from build123d import *

# Parameters (mm, degrees)
ESBO_O1_W                  = 44
ESBO_O1_H                  = 44
RESSALTO_EXTRUS_O1_DEPTH   = 12
ESBO_O2_R                  = 18
RESSALTO_EXTRUS_O2_DEPTH   = 17
CHANFRO1_SIZE              = 7
CORTE_EXTRUS_O1_DEPTH      = 1
CORTE_EXTRUS_O1_DEPTH_BACK = 43.532340636
ESBO_O3_R                  = 6
ESBO_O3_R_2                = 2.5
ESBO_O4_R                  = 4
CORTE_EXTRUS_O2_DEPTH      = 5
CHANFRO2_SIZE              = 0.5
CHANFRO3_SIZE              = 0.5
ESBO_O5_R                  = 7.5
ESBO_O5_R_2                = 7.25
CORTE_EXTRUS_O3_DEPTH      = 1
ESBO_O6_R                  = 8.146724453
ESBO_O6_R_2                = 7.952420513
CORTE_EXTRUS_O4_DEPTH      = 1
ESBO_O7_R                  = 12.470388764
ESBO_O7_R_2                = 11.825568989
CORTE_EXTRUS_O5_DEPTH      = 1
FILETE1_R                  = 0.2
FILETE2_R                  = 0.2


with BuildPart() as part:
    # Esboço1 → Ressalto-extrusão1 (new body)
    with BuildSketch(Plane.XY):
        Rectangle(ESBO_O1_W, ESBO_O1_H)
    extrude(amount=RESSALTO_EXTRUS_O1_DEPTH)

    # Esboço2 → Ressalto-extrusão2 (add)
    with BuildSketch(Plane(origin=(0, 0, 0), x_dir=(-1, 0, 0), z_dir=(0, 0, -1))):
        with Locations(Location((0, 0, 0), (0, 0, 180))):
            Circle(ESBO_O2_R)
    extrude(amount=RESSALTO_EXTRUS_O2_DEPTH)

    # Chanfro1
    chanfro1_edges = [part.edges().sort_by_distance(p)[0] for p in [
        (-22, 22, 6),
        (22, 22, 6),
        (22, -22, 6),
        (-22, -22, 6),
    ]]
    chamfer(chanfro1_edges, length=CHANFRO1_SIZE)

    # Esboço3 → Corte-extrusão1 (cut, two sides: drawn at the far end of the back side and taken through both)
    with BuildSketch(Plane.XY.offset(12).offset(-CORTE_EXTRUS_O1_DEPTH_BACK)):
        Circle(ESBO_O3_R)
        with Locations((-15.5, 15.5)):
            Circle(ESBO_O3_R_2)
        with Locations((15.5, 15.5)):
            Circle(ESBO_O3_R_2)
        with Locations((15.5, -15.5)):
            Circle(ESBO_O3_R_2)
        with Locations((-15.5, -15.5)):
            Circle(ESBO_O3_R_2)
    extrude(amount=CORTE_EXTRUS_O1_DEPTH + CORTE_EXTRUS_O1_DEPTH_BACK, mode=Mode.SUBTRACT)

    # Esboço4 → Corte-extrusão2 (cut)
    with BuildSketch(Plane.XY.offset(12)):
        with Locations((-15.5, 15.5)):
            Circle(ESBO_O4_R)
        with Locations((15.5, 15.5)):
            Circle(ESBO_O4_R)
        with Locations((15.5, -15.5)):
            Circle(ESBO_O4_R)
        with Locations((-15.5, -15.5)):
            Circle(ESBO_O4_R)
    extrude(amount=-CORTE_EXTRUS_O2_DEPTH, mode=Mode.SUBTRACT)

    # Chanfro2
    # the kernel refuses this chamfer: 0.5 mm, written as the material it takes off along each edge
    with BuildSketch(Plane(origin=(0, 0, -17), x_dir=(1, 0, 0), z_dir=(0, 1, 0))) as chanfro2_piece_1:
        Polygon((18, -CHANFRO2_SIZE), (18 - CHANFRO2_SIZE, 0), (18, 0), align=None)
    revolve(axis=Axis((0, 0, -17), (0, 0, -1)), mode=Mode.SUBTRACT)
    with BuildSketch(Plane(origin=(16.285841494, -22, 12), x_dir=(0, 0.9996219169112968, 0.02749587661058555), z_dir=(-1, 0, 0)), Plane(origin=(-22, -16.285841494, 12), x_dir=(0.9996219169112968, 0, 0.02749587661058555), z_dir=(0, 1, 0)), Plane(origin=(22, 16.285841494, 12), x_dir=(-0.9996219169112968, 0, 0.02749587661058555), z_dir=(0, -1, 0))) as chanfro2_piece_2:
        Polygon((CHANFRO2_SIZE * 0.999621916911, CHANFRO2_SIZE * 0.0274958766106), (-CHANFRO2_SIZE * 0.0274958766106, CHANFRO2_SIZE * 0.999621916911), (0, 0), align=None)
    extrude(amount=32.571682988, mode=Mode.SUBTRACT)
    with BuildSketch(Plane(origin=(-16.285841494, 22, 12), x_dir=(0, 0.0274958766105891, -0.9996219169112968), z_dir=(1, 0, 0))) as chanfro2_piece_3:
        Polygon((CHANFRO2_SIZE * 0.999621916911, -CHANFRO2_SIZE * 0.0274958766106), (-CHANFRO2_SIZE * 0.0274958766106, -CHANFRO2_SIZE * 0.999621916911), (0, 0), align=None)
    extrude(amount=32.571682988, mode=Mode.SUBTRACT)
    with BuildSketch(Plane(origin=(-14.09077276, 22.90922724, 12), x_dir=(-0.019442520806015533, 0.019442520806015533, -0.9996219169112968), z_dir=(-0.7071067811865476, -0.7071067811865476, 0)), Plane(origin=(22.90922724, -14.09077276, 12), x_dir=(-0.7068394360706735, 0.7068394360706735, 0.02749587661058563), z_dir=(-0.7071067811865476, -0.7071067811865476, 0))) as chanfro2_piece_4:
        Polygon((CHANFRO2_SIZE * 0.999621916911, CHANFRO2_SIZE * 0.0274958766106), (-CHANFRO2_SIZE * 0.0274958766106, CHANFRO2_SIZE * 0.999621916911), (0, 0), align=None)
    extrude(amount=12.471177925, mode=Mode.SUBTRACT)
    with BuildSketch(Plane(origin=(14.09077276, 22.90922724, 12), x_dir=(0.019442520806015533, 0.019442520806015533, -0.9996219169112968), z_dir=(0.7071067811865476, -0.7071067811865476, 0)), Plane(origin=(-22.90922724, -14.09077276, 12), x_dir=(0.7068394360706735, 0.7068394360706735, 0.02749587661058563), z_dir=(0.7071067811865476, -0.7071067811865476, 0))) as chanfro2_piece_5:
        Polygon((CHANFRO2_SIZE * 0.999621916911, -CHANFRO2_SIZE * 0.0274958766106), (-CHANFRO2_SIZE * 0.0274958766106, -CHANFRO2_SIZE * 0.999621916911), (0, 0), align=None)
    extrude(amount=12.471177925, mode=Mode.SUBTRACT)
    with BuildSketch(Plane(origin=(0, 0, 12), x_dir=(1, 0, 0), z_dir=(0, -1, 0))) as chanfro2_piece_6:
        Polygon((6 + CHANFRO2_SIZE, 0), (6, -CHANFRO2_SIZE), (6, 0), align=None)
    revolve(axis=Axis((0, 0, 12), (0, 0, 1)), mode=Mode.SUBTRACT)
    with BuildSketch(Plane(origin=(0, 0, -17), x_dir=(1, 0, 0), z_dir=(0, -1, 0))) as chanfro2_piece_7:
        Polygon((6, CHANFRO2_SIZE), (6 + CHANFRO2_SIZE, 0), (6, 0), align=None)
    revolve(axis=Axis((0, 0, -17), (0, 0, 1)), mode=Mode.SUBTRACT)
    with BuildSketch(Plane(origin=(-15.5, 15.5, 12), x_dir=(1, 0, 0), z_dir=(0, -1, 0))) as chanfro2_piece_8:
        Polygon((4 + CHANFRO2_SIZE, 0), (4, -CHANFRO2_SIZE), (4, 0), align=None)
    revolve(axis=Axis((-15.5, 15.5, 12), (0, 0, 1)), mode=Mode.SUBTRACT)
    with BuildSketch(Plane(origin=(15.5, 15.5, 12), x_dir=(1, 0, 0), z_dir=(0, -1, 0))) as chanfro2_piece_9:
        Polygon((4 + CHANFRO2_SIZE, 0), (4, -CHANFRO2_SIZE), (4, 0), align=None)
    revolve(axis=Axis((15.5, 15.5, 12), (0, 0, 1)), mode=Mode.SUBTRACT)
    with BuildSketch(Plane(origin=(15.5, -15.5, 12), x_dir=(1, 0, 0), z_dir=(0, -1, 0))) as chanfro2_piece_10:
        Polygon((4 + CHANFRO2_SIZE, 0), (4, -CHANFRO2_SIZE), (4, 0), align=None)
    revolve(axis=Axis((15.5, -15.5, 12), (0, 0, 1)), mode=Mode.SUBTRACT)
    with BuildSketch(Plane(origin=(-15.5, -15.5, 12), x_dir=(1, 0, 0), z_dir=(0, -1, 0))) as chanfro2_piece_11:
        Polygon((4 + CHANFRO2_SIZE, 0), (4, -CHANFRO2_SIZE), (4, 0), align=None)
    revolve(axis=Axis((-15.5, -15.5, 12), (0, 0, 1)), mode=Mode.SUBTRACT)

    # Chanfro3
    chanfro3_edges = [part.edges().sort_by_distance(p)[0] for p in [
        (0, -22, 0),
        (-22, 0, 0),
        (0, 22, 0),
        (22, 0, 0),
        (-18.5, 18.5, 0),
        (18.5, 18.5, 0),
        (18.5, -18.5, 0),
        (-18.5, -18.5, 0),
    ]]
    chamfer(chanfro3_edges, length=CHANFRO3_SIZE)

    # Esboço5 → Corte-extrusão3 (cut)
    with BuildSketch(Plane(origin=(0, 0, -17), x_dir=(-1, 0, 0), z_dir=(0, 0, -1))):
        Circle(ESBO_O5_R)
        Circle(ESBO_O5_R_2, mode=Mode.SUBTRACT)
    corte_extrus_o3 = extrude(amount=-CORTE_EXTRUS_O3_DEPTH, mode=Mode.SUBTRACT)

    # Esboço6 → Corte-extrusão4 (cut)
    with BuildSketch(Plane(origin=(0, 0, -17), x_dir=(-1, 0, 0), z_dir=(0, 0, -1))):
        Circle(ESBO_O6_R)
        Circle(ESBO_O6_R_2, mode=Mode.SUBTRACT)
    corte_extrus_o4 = extrude(amount=-CORTE_EXTRUS_O4_DEPTH, mode=Mode.SUBTRACT)

    # Esboço7 → Corte-extrusão5 (cut)
    with BuildSketch(Plane(origin=(0, 0, -17), x_dir=(-1, 0, 0), z_dir=(0, 0, -1))):
        Circle(ESBO_O7_R)
        Circle(ESBO_O7_R_2, mode=Mode.SUBTRACT)
    corte_extrus_o5 = extrude(amount=-CORTE_EXTRUS_O5_DEPTH, mode=Mode.SUBTRACT)

    # Filete1
    filete1_edges = [part.edges().sort_by_distance(p)[0] for p in [
        (7.5, 0, -17),
        (7.952420513, 0, -17),
    ]]
    fillet(filete1_edges, radius=FILETE1_R)

    # Espelhar3: Corte-extrusão3, Corte-extrusão4, Corte-extrusão5 across plane
    add(corte_extrus_o3.mirror(Plane.XY.offset(-2.5)), mode=Mode.SUBTRACT)
    add(corte_extrus_o4.mirror(Plane.XY.offset(-2.5)), mode=Mode.SUBTRACT)
    add(corte_extrus_o5.mirror(Plane.XY.offset(-2.5)), mode=Mode.SUBTRACT)

    # Filete2
    filete2_edges = [part.edges().sort_by_distance(p)[0] for p in [
        (7.5, 0, 12),
        (7.952420513, 0, 12),
    ]]
    fillet(filete2_edges, radius=FILETE2_R)


solid = part.part
For this review, take the finished solid that the model builds, in its own axes (mm). A direction names the side the tool comes from. Round coordinates to 2 decimals unless told otherwise and drop trailing zeros. Loops run counter-clockwise (first coordinate to the right, second up) from the corner with the lowest first, then second, coordinate; pieces in that order, holes last. Notation, with made-up numbers: (46.25, 38.25) - (90.25, 38.25) arc R32 ccw to (90.25, 64.25) - close; hole circle Ø8 at (-16.5, 83). An arc over 180 degrees is marked (long way). Put each result on its own line as item: value. Start each with the question number.
1. For faces 1 (the cylindrical face through (-7.77, 2.45, -16.51)), 2 (the cylindrical face through (2.703, -12.174, 11.507)), 3 (the flat face through (-3, 8, -17)), list the 3-axis set-ups (+Z, -Z, +X, -X, +Y, -Y) from which the entire face can be reached by the end or side of a thin tool; tool diameter is ignored.
2. Consider section B-B on y = -14. State how many separate pieces and enclosed holes the cut face has, plus the area to 3 significant figures.
3. Consider section A-A on z = -0.75. State the section outline as (x, y) points, plus the area to 3 significant figures.
4. Insertion check: P1, Ø2, axis at x = 10.5, z = -11, coming from the +Y side; P2, Ø12.5, axis at x = -0.5, y = -5, coming from the +Z side; P3, Ø3, axis at y = 14, z = -8, coming from the +X side; P4, Ø6.5, axis at x = 15.5, y = -15.5, coming from the -Z side. Each pin has a flat end and moves straight along its axis. Give the tip position at first contact, or say it passes through.
5. Mouldability with a two-part tool opening along Y and no side actions: class faces 4 (the flat face through (-14.43, -11.05, 0)), 5 (the cylindrical face through (7.493, 0.33, -16.406)), 6 (the flat face through (18.28, -18.37, 0.25)) as +Y half, -Y half, draft (parallel to the pull), parting line (faces both ways), or undercut.
6. For probe 1 along Y at (x, z) = (-15.5, 8); probe 2 along Y at (x, z) = (-1.5, -1.25); probe 3 along X at (y, z) = (-5, 1), list the stretches that pass through material, from the lowest coordinate up. Write a range as [from, to].
Result sheet:
1. face 1: -Z
1. face 2: +Z
1. face 3: -Z, +X, -X, +Y, -Y
2. separate pieces: 3
2. enclosed holes: 0
2. area: 781 mm^2
3. outline: circle Ø36 at (0, 0); hole circle Ø12 at (0, 0)
3. area: 905 mm^2
4. P1: y = 15.29
4. P2: z = 12
4. P3: x = 12.95
4. P4: z = 0
5. face 4: draft
5. face 5: undercut
5. face 6: -Y half
6. probe 1: [-21.5, -19.5], [-11.5, 11.5], [19.5, 21.5]
6. probe 2: [-17.94, -5.81], [5.81, 17.94]
6. probe 3: [-22, -3.32], [3.32, 22]
